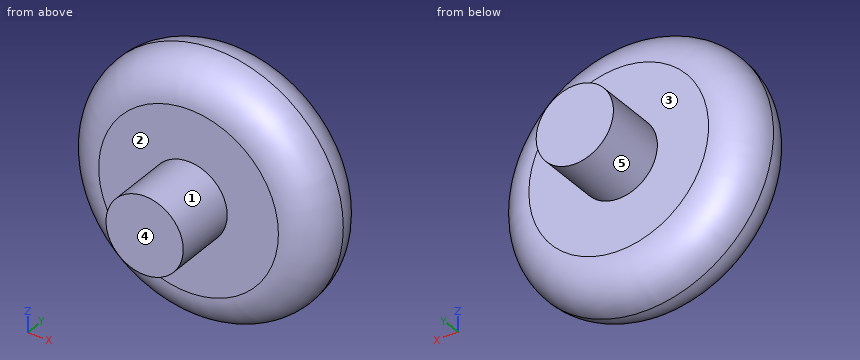
from build123d import *

# Parameters (mm, degrees)
F0_R     = 15.046961384
F1_DEPTH = 40
F0_R_2   = 50
F2_DEPTH = 15
F3_R     = 14.99999


# Not quite as in the source:
# - a fillet or chamfer is up to 0.001 mm smaller than in the source, because OpenCascade refuses the exact size


with BuildPart() as f1:
    # F0 (on Front) → F1 (new body, symmetric)
    with BuildSketch(Plane.XZ):
        Circle(F0_R)
    extrude(amount=F1_DEPTH, both=True)

    # F0 (on Front) → F2 (join, symmetric)
    with BuildSketch(Plane.XZ):
        Circle(F0_R_2)
        Circle(F0_R, mode=Mode.SUBTRACT)
    extrude(amount=F2_DEPTH, both=True)

    # F3 (radius 15 in the source; OpenCascade refuses exactly that, so slightly less here)
    f3_edges = [f1.edges().sort_by_distance(p)[0] for p in [
        (-50, -15, 0),
        (-50, 15, 0),
    ]]
    fillet(f3_edges, radius=F3_R)


solid = f1.part
The listing builds one solid part. Answer for the finished solid, in the listing's coordinates (mm). Face numbers are marked on the shaded views. A direction names the side the tool comes from. Coordinates: 2 decimals unless noted, no trailing zeros. Write each loop counter-clockwise with the first axis right and the second up, starting at its lowest first coordinate (ties: lowest second). Pieces come first, ordered by that corner, then holes. Notation, with made-up numbers: (54.25, 41) - (78.25, 41) arc R22 ccw to (78.25, 71) - close; hole circle Ø4 at (79, 33). An arc over 180 degrees is marked (long way). Put each result on its own line as item: value.
1. Find the intervals of material crossed by line 1 along Y through (x, z) = (24.5, 4.5); line 2 along Z through (x, y) = (-11, -8); line 3 along X through (y, z) = (11, -32), in increasing order. Write a range as from..to.
Answer sheet:
line 1: y = -15..15
line 2: z = -46.4..46.4
line 3: x = -31.92..31.92
2. Flat-ended cylindrical pins translate along their axes: pin 1 Ø10 at (x, y) = (10.5, 26.5) entering from +Z; pin 2 Ø5 at (x, z) = (17.5, 28) entering from +Y; pin 3 Ø4 at (x, y) = (-38, 11.5) entering from -Z. Find the tip coordinate at first contact, or state that the pin passes through.
Answer sheet:
pin 1: stops at z = 14.01
pin 2: stops at y = 15
pin 3: stops at z = -28.06
3. The part is cut by section C-C on y = 9. Give the vertices of the cut face in (x, z), plus the area to 3 significant figures.
Answer sheet:
outline: circle Ø94 at (0, 0)
area: 6,940 mm^2
4. A tool of negligible diameter and unlimited length cuts with its end or side. For the marked faces 4 and 5, from which of +Z, -Z, +X, -X, +Y, -Y can it reach the whole face along a straight path? Write none if from no direction.
Answer sheet:
face 4: +Z, -Z, +X, -X, -Y
face 5: +Y
5. Determine the mould class of the marked faces 1, 2 and 3 for opening direction Y: pulls with the +Y half, pulls with the -Y half, needs draft (parallel to the pull), parting line crosses it, or undercut.
Answer sheet:
face 1: needs draft
face 2: pulls with the -Y half
face 3: pulls with the +Y half
